Check sheet for the modelled part. Datum: model origin and axes. Units: mm. A direction names the side the tool comes from. Coordinates: 2 decimals unless noted, no trailing zeros. Loops run counter-clockwise (first coordinate to the right, second up) from the corner with the lowest first, then second, coordinate; pieces in that order, holes last.
```python
from build123d import *

# Parameters (mm, degrees)
SKETCH1_W           = 50.8
SKETCH1_H           = 50.8
SKETCH1_R           = 5.3721
BOSS_EXTRUDE1_DEPTH = 25.4
SKETCH2_W           = 50.8
SKETCH2_H           = 25.4
CUT_EXTRUDE1_DEPTH  = 6.35
SKETCH3_R           = 4.7625
CUT_EXTRUDE2_DEPTH  = 12.7


with BuildPart() as part:
    # Sketch1 → Boss-Extrude1 (new body)
    with BuildSketch(Plane(origin=(0, 0, 0), x_dir=(0, 0, -1), z_dir=(1, 0, 0))):
        Rectangle(SKETCH1_W, SKETCH1_H)
        with Locations((0, -9.525)):
            Circle(SKETCH1_R, mode=Mode.SUBTRACT)
    extrude(amount=BOSS_EXTRUDE1_DEPTH)

    # Sketch2 → Cut-Extrude1 (cut)
    with BuildSketch(Plane.ZY):
        with Locations((0, 12.7)):
            Rectangle(SKETCH2_W, SKETCH2_H)
    extrude(amount=-CUT_EXTRUDE1_DEPTH, mode=Mode.SUBTRACT)

    # Sketch3 → Cut-Extrude2 (cut)
    with BuildSketch(Plane.ZY.offset(-6.35)):
        with Locations((0, 12.7)):
            Circle(SKETCH3_R)
    extrude(amount=-CUT_EXTRUDE2_DEPTH, mode=Mode.SUBTRACT)


solid = part.part
```
1) Section check A-A on z = 0. Enter the section's corners in (x, y).
Answer sheet:
outline: (0, -25.4) - (25.4, -25.4) - (25.4, -14.9) - (0, -14.9) - close; (0, -4.15) - (25.4, -4.15) - (25.4, 25.4) - (6.35, 25.4) - (6.35, 17.46) - (19.05, 17.46) - (19.05, 7.94) - (6.35, 7.94) - (6.35, 0) - (0, 0) - close
2) Scan lines: line 1 (Y direction, x = 11.25, z = 0); line 2 (X direction, y = 22, z = 19); line 3 (Z direction, x = 16, y = -11). Record each from-to range of solid material in increasing order.
Answer sheet:
line 1: y = -25.4 to -14.9, -4.15 to 7.94, 17.46 to 25.4
line 2: x = 6.35 to 25.4
line 3: z = -25.4 to -5.17, 5.17 to 25.4
3) Section check C-C on x = 21.75. Enter the section's corners in (y, z) (3 decimals).
Answer sheet:
outline: (-25.4, -25.4) - (25.4, -25.4) - (25.4, 25.4) - (-25.4, 25.4) - close; hole circle Ø10.744 at (-9.525, 0)
4) Mould release check, pull along Y, two halves, no side actions. Record for faces 1 (the flat face through (13, 0, 25.4)), 2 (the cylindrical face through (12.61, 8.05, -1.03)), 3 (the flat face through (3, 0, 0)): +Y half, -Y half, draft (parallel to the pull), parting line (faces both ways), or undercut.
Answer sheet:
face 1: draft
face 2: undercut
face 3: +Y half
5) Section check B-B on y = 12.7. Enter the section's corners in (x, z), plus the area to 3 significant figures.
Answer sheet:
outline: (6.35, -25.4) - (25.4, -25.4) - (25.4, 25.4) - (6.35, 25.4) - (6.35, 4.76) - (19.05, 4.76) - (19.05, -4.76) - (6.35, -4.76) - close
area: 847 mm2
6) Section check D-D on y = -13. Enter the section's corners in (x, z).
Answer sheet:
outline: (0, -25.4) - (25.4, -25.4) - (25.4, -4.1) - (0, -4.1) - close; (0, 4.1) - (25.4, 4.1) - (25.4, 25.4) - (0, 25.4) - close
7) Depth check by flat-ended pin: pin 1 (5 mm diameter, centred on y = 12.5, z = 0, fed in from -X); pin 2 (1.9 mm diameter, centred on x = 2, z = -3.5, fed in from +Y); pin 3 (20.5 mm diameter, centred on y = 18.5, z = -5, fed in from -X). Enter the tip coordinate at first touch or a pass-through.
Answer sheet:
pin 1: stops at x = 19.05
pin 2: stops at y = 0
pin 3: stops at x = 6.35
8) Set-up check for faces 4 (the flat face through (6.35, 13, 5)), 5 (the flat face through (19.05, 13, 0)), 6 (the flat face through (13, 0, -25.4)): record each of +Z, -Z, +X, -X, +Y, -Y from which the full face is reachable in a straight line by a thin tool's end or side.
Answer sheet:
face 4: +Z, -Z, -X, +Y
face 5: -X
face 6: -Z, +X, -X, +Y, -Y
